Check sheet for the drawn part. Datum: minimum x, y, z corner. Units: mm. Coordinates: 2 decimals unless noted, no trailing zeros. Write each loop counter-clockwise with the first axis right and the second up, starting at its lowest first coordinate (ties: lowest second). Pieces come first, ordered by that corner, then holes. Notation, with made-up numbers: (50, 87.5) -> (82, 87.5) arc R23 cw to (82, 118.5) -> close; hole circle Ø1 at (72.5, 15.25). An arc over 180 degrees is marked (long way). Answer in a Markdown table with one row per item. Add a question column.
1. Cross-section at C-C on x = 0.5. Record the cut outline in (y, z), and give its area (3 significant figures).
2. Scan lines: L1, parallel to Y at x = 1.25, z = 3.25; L2, parallel to X at y = 2.25, z = 5.5; L3, parallel to Y at x = 1.95, z = 0.5. Record each from-to range of solid material in increasing order. Write a range as from..to.
3. Cross-section at A-A on x = 1.25. Record the cut outline in (y, z), and give its area (3 significant figures).
4. Cross-section at D-D on x = 1.65. Record the cut outline in (y, z).
5. Cross-section at B-B on z = 8.25. Record the cut outline in (x, y).
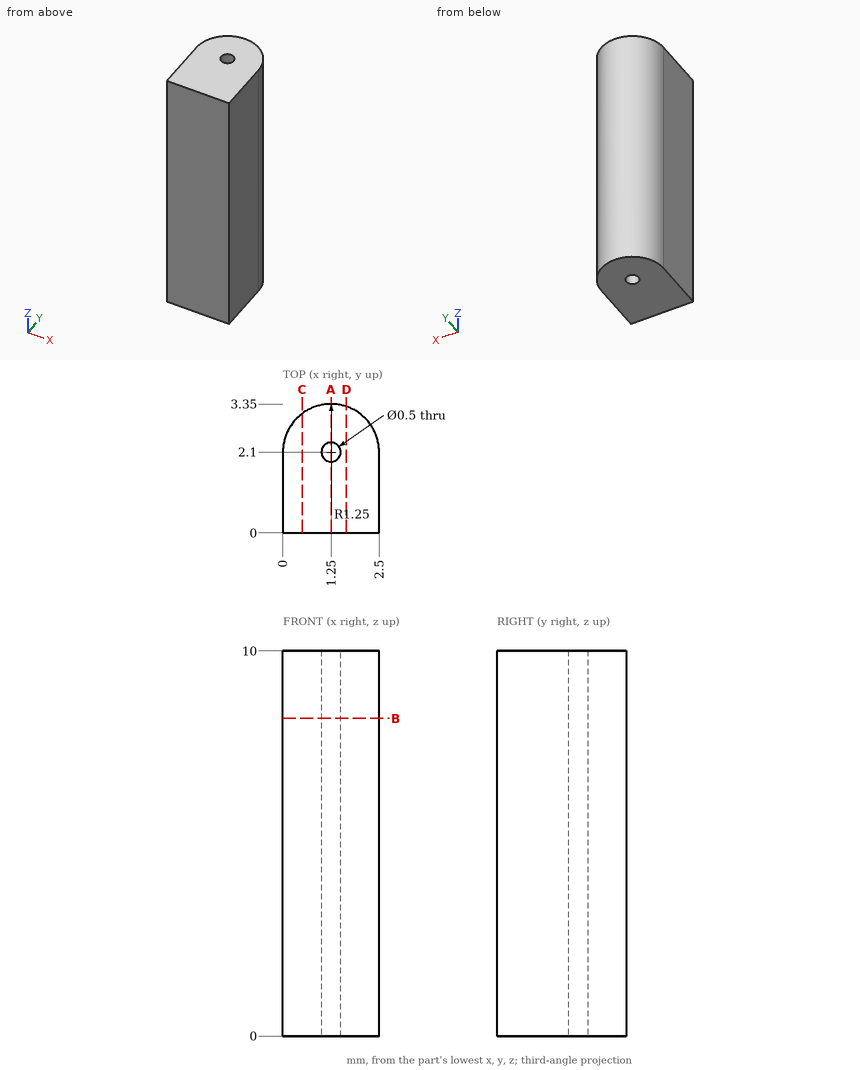
Results found:
| question | item | result |
|---|---|---|
| 1 | outline | (0, 0) -> (3.1, 0) -> (3.1, 10) -> (0, 10) -> close |
| 1 | area | 31.0 mm^2 |
| 2 | L1 | y = 0..1.85, 2.35..3.35 |
| 2 | L2 | x = 0.01..1.05, 1.45..2.49 |
| 2 | L3 | y = 0..3.14 |
| 3 | outline | (0, 0) -> (1.85, 0) -> (1.85, 10) -> (0, 10) -> close; (2.35, 0) -> (3.35, 0) -> (3.35, 10) -> (2.35, 10) -> close |
| 3 | area | 28.5 mm^2 |
| 4 | outline | (0, 0) -> (3.28, 0) -> (3.28, 10) -> (0, 10) -> close |
| 5 | outline | (0, 0) -> (2.5, 0) -> (2.5, 2.1) arc R1.25 ccw to (0, 2.1) -> close; hole circle Ø0.5 at (1.25, 2.1) |
